Autodesk Inventor part; units mm, degrees
ref_plane "YZ Plane" through (0, 0, 0) normal (1, 0, 0) x (0, 1, 0)
ref_plane "XZ Plane" through (0, 0, 0) normal (0, 1, 0) x (-1, 0, 0)
ref_plane "XY Plane" through (0, 0, 0) normal (0, 0, 1) x (1, 0, 0)
sketch "Sketch1" plane through (0, 0, 0) normal (0, 1, 0) x (-1, 0, 0)
  line L0 (0, 0) -> (12.5, 0)
  circle A0 centre (12.5, 0) radius 9.65
  circle A1 centre (12.5, 0) radius 12.5
  line L1 (12.5, 12.5) -> (-1, 12.5)
  line L2 (-1, 12.5) -> (-1, -12.5)
  line L3 (-1, -12.5) -> (12.5, -12.5)
  circle A2 centre (12.5, 0) radius 8
  line L4 (-1, -12.5) -> (4, -12.5)
  line L5 (4, -12.5) -> (4, -22.5)
  line L6 (4, -22.5) -> (-1, -22.5)
  line L7 (-1, -22.5) -> (-1, -12.5)
  line L8 (-1, 12.5) -> (-1, 22.5)
  line L9 (-1, 22.5) -> (4.5, 22.5)
  line L10 (4.5, 22.5) -> (4.5, 12.5)
  dimension "d0" = 12.5
  dimension "d1" = 19.3
  dimension "d2" = 16
  dimension "d7" = 5
  dimension "d8" = 10
  dimension "d9" = 10
extrude "Extrusion3" add sketch "Sketch1" along normal blind 3 contours A0
extrude "Extrusion4" add sketch "Sketch1" along normal blind 9 contours A1 L3 L2 L1 | A1 | L1 L8 L9 L10 | L5 L6 L7 L3
sketch "Sketch4" plane through (1, 0, 22.5) normal (1, 0, 0) x (0, 0, -1)
  line L0 (0, 0) -> (0, 9)
  line L1 (0, 4.5) -> (5, 4.5)
  line L2 (45, 0) -> (45, 9)
  line L3 (45, 4.5) -> (40, 4.5)
  circle A0 centre (5, 4.5) radius 2.55
  circle A1 centre (40, 4.5) radius 2.55
  point P0 (22.5, 0)
  dimension "d14" = 5
  dimension "d15" = 5
  dimension "d16" = 5.1
  dimension "d17" = 5.1
extrude "Extrusion5" cut sketch "Sketch4" against normal blind 7
properties part number "wheel_shaft_holder_small"
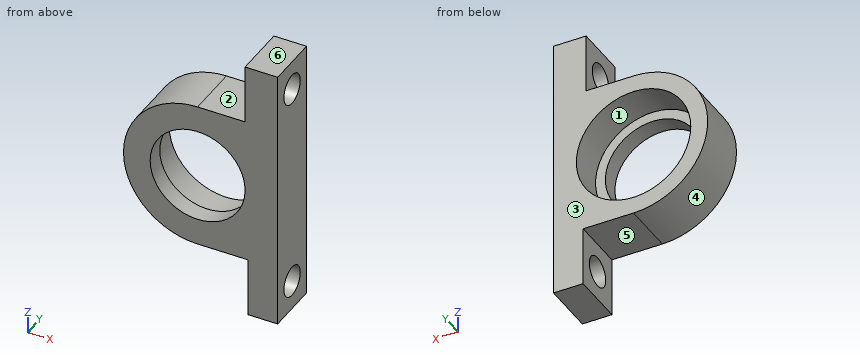
The listing builds one solid part. Answer for the finished solid, in the listing's coordinates (mm). Face numbers are marked on the shaded views. A direction names the side the tool comes from. Give positions to 0.01 mm unless a question says otherwise; leave off trailing zeros. Write each loop counter-clockwise with the first axis right and the second up, starting at its lowest first coordinate (ties: lowest second). Pieces come first, ordered by that corner, then holes. Notation, with made-up numbers: (-2, -29.5) -> (12, -29.5) arc R19 cw to (12, -20.5) -> close; hole circle Ø3 at (-12, 39). An arc over 180 degrees is marked (long way). Use a Markdown table: item, result.
(1) Determine the mould class of the marked faces 1, 2, 3 and 4 for opening direction Z: released by +Z, released by -Z, zero draft, split by the parting line, or undercut.
Return value:
| item | result |
|---|---|
| face 1 | undercut |
| face 2 | released by +Z |
| face 3 | zero draft |
| face 4 | split by the parting line |
(2) Section B-B, the plane y = 8.5 is taken. Determine the outline of the cut face in (x, z).
Return value:
| item | result |
|---|---|
| outline | (-12.5, -12.5) -> (-4, -12.5) -> (-4, -22.5) -> (1, -22.5) -> (1, 22.5) -> (-4.5, 22.5) -> (-4.5, 12.5) -> (-12.5, 12.5) arc R12.5 ccw to start; hole circle Ø19.3 at (-12.5, 0) |
(3) Flat-ended cylindrical pins translate along their axes: P1, Ø6, axis at x = -17, z = -3, coming from the +Y side; P2, Ø5, axis at x = -7.5, y = 7.5, coming from the -Z side. Find the tip coordinate at first contact, or state that the pin passes through.
Return value:
| item | result |
|---|---|
| P1 | y = 3 |
| P2 | z = -12.5 |
(4) For the marked faces 5 and 6, determine the directions among +Z, -Z, +X, -X, +Y, -Y from which every point of the face is accessible in a straight line to the end or side of a thin tool.
Return value:
| item | result |
|---|---|
| face 5 | -Z, -X, +Y, -Y |
| face 6 | +Z, +X, -X, +Y, -Y |
(5) Find the intervals of material crossed by probe 1 along Y at (x, z) = (-2.3, -17.5); probe 2 along X at (y, z) = (6.7, 0); probe 3 along X at (y, z) = (4, -13), in increasing order. Write a range as from..to.
Return value:
| item | result |
|---|---|
| probe 1 | 0..1.95, 7.05..9 |
| probe 2 | -25..-22.15, -2.85..1 |
| probe 3 | -4..1 |
(6) Section A-A, the plane z = -17.5 is taken. Determine the outline of the cut face in (x, y).
Return value:
| item | result |
|---|---|
| outline | (-4, 0) -> (1, 0) -> (1, 1.95) -> (-4, 1.95) -> close; (-4, 7.05) -> (1, 7.05) -> (1, 9) -> (-4, 9) -> close |
(7) Section D-D, the plane x = -11 is taken. Determine the outline of the cut face in (y, z).
Return value:
| item | result |
|---|---|
| outline | (0, -12.5) -> (9, -12.5) -> (9, -9.53) -> (3, -9.53) -> (3, -7.86) -> (0, -7.86) -> close; (0, 7.86) -> (3, 7.86) -> (3, 9.53) -> (9, 9.53) -> (9, 12.5) -> (0, 12.5) -> close |
(8) Section C-C, the plane y = 4.5 is taken. Determine the outline of the cut face in (x, z).
Return value:
| item | result |
|---|---|
| outline | (-12.5, -12.5) -> (-4, -12.5) -> (-4, -14.95) -> (1, -14.95) -> (1, 14.95) -> (-4.5, 14.95) -> (-4.5, 12.5) -> (-12.5, 12.5) arc R12.5 ccw to start; (-4.5, 20.05) -> (1, 20.05) -> (1, 22.5) -> (-4.5, 22.5) -> close; (-4, -22.5) -> (1, -22.5) -> (1, -20.05) -> (-4, -20.05) -> close; hole circle Ø19.3 at (-12.5, 0) |
